from build123d import *

# Parameters (mm, degrees)
SKETCH1_W           = 110
SKETCH1_H           = 48
SKETCH1_R           = 2.1
BOSS_EXTRUDE1_DEPTH = 1.5
FILLET1_R           = 1.5


with BuildPart() as part:
    # Sketch1 → Boss-Extrude1 (new body, symmetric)
    with BuildSketch(Plane.XY):
        Rectangle(SKETCH1_W, SKETCH1_H)
        with Locations((50, 9)):
            Circle(SKETCH1_R, mode=Mode.SUBTRACT)
        with Locations((26, 9)):
            Circle(SKETCH1_R, mode=Mode.SUBTRACT)
        with Locations((50, -9)):
            Circle(SKETCH1_R, mode=Mode.SUBTRACT)
        with Locations((26, -9)):
            Circle(SKETCH1_R, mode=Mode.SUBTRACT)
        with Locations((-50, 9)):
            Circle(SKETCH1_R, mode=Mode.SUBTRACT)
        with Locations((-26, 9)):
            Circle(SKETCH1_R, mode=Mode.SUBTRACT)
        with Locations((-50, -9)):
            Circle(SKETCH1_R, mode=Mode.SUBTRACT)
        with Locations((-26, -9)):
            Circle(SKETCH1_R, mode=Mode.SUBTRACT)
        with Locations((-38, 19.5)):
            Circle(SKETCH1_R, mode=Mode.SUBTRACT)
        with Locations((-38, -19.5)):
            Circle(SKETCH1_R, mode=Mode.SUBTRACT)
        with Locations((38, 19.5)):
            Circle(SKETCH1_R, mode=Mode.SUBTRACT)
        with Locations((38, -19.5)):
            Circle(SKETCH1_R, mode=Mode.SUBTRACT)
        with Locations((12.5, -9)):
            Circle(SKETCH1_R, mode=Mode.SUBTRACT)
        with Locations((-12.5, -9)):
            Circle(SKETCH1_R, mode=Mode.SUBTRACT)
        with Locations((-12.5, 7)):
            Circle(SKETCH1_R, mode=Mode.SUBTRACT)
        with Locations((12.5, 7)):
            Circle(SKETCH1_R, mode=Mode.SUBTRACT)
    extrude(amount=BOSS_EXTRUDE1_DEPTH, both=True)

    # Fillet1
    fillet1_edges = [part.edges().sort_by_distance(p)[0] for p in [
        (-55, 24, 0),
        (55, 24, 0),
        (55, -24, 0),
        (-55, -24, 0),
    ]]
    fillet(fillet1_edges, radius=FILLET1_R)


solid = part.part
The listing builds one solid part. Answer for the finished solid, in the listing's coordinates (mm). Coordinates: 2 decimals unless noted, no trailing zeros. Loops run counter-clockwise (first coordinate to the right, second up) from the corner with the lowest first, then second, coordinate; pieces in that order, holes last. Notation, with made-up numbers: (81.5, 26) -> (106.5, 26) arc R22 ccw to (106.5, 55) -> close; hole circle Ø4 at (19, 32.25). An arc over 180 degrees is marked (long way). Answer in a Markdown table with one row per item. Add a question column.
1. The part is cut by section D-D, the plane z = 0. Count the separate pieces of the cut face and the enclosed holes in it, then the cut area to 3 significant figures.
2. A flat-ended cylindrical pin translates along its axis: P1, Ø3.5, axis at x = 12.5, y = -9, coming from the +Z side. Find the tip coordinate at first contact, or state that the pin passes through.
3. Consider line 1 (Y direction, x = 26, z = 0.85); line 2 (Y direction, x = -12.5, z = 0.7); line 3 (X direction, y = -21, z = -1.2). Determine where each line is inside the solid, lowest interval first. Write a range as [from, to].
4. The part is cut by section C-C, the plane y = -19.5. Write down the section's boundary in (x, z).
5. Determine the mould class of faces 1 (the cylindrical face through (12.227, -6.918, -0.021)), 2 (the flat face through (55, 0, 0)), 3 (the flat face through (-1, 24, 0)), 4 (the cylindrical face through (36.452, -18.081, -0.021)) for opening direction X: +X half, -X half, draft (parallel to the pull), parting line (faces both ways), or undercut.
6. The part is cut by section A-A, the plane y = -9. Write down the section's boundary in (x, z).
7. The part is cut by section B-B, the plane x = -50. Write down the section's boundary in (y, z), then the cut area to 3 significant figures.
Answer below:
| question | item | result |
|---|---|---|
| 1 | separate pieces | 1 |
| 1 | enclosed holes | 16 |
| 1 | area | 5,060 mm2 |
| 2 | P1 | through |
| 3 | line 1 | [-24, -11.1], [-6.9, 6.9], [11.1, 24] |
| 3 | line 2 | [-24, -11.1], [-6.9, 4.9], [9.1, 24] |
| 3 | line 3 | [-55, -39.47], [-36.53, 36.53], [39.47, 55] |
| 4 | outline | (-55, -1.5) -> (-40.1, -1.5) -> (-40.1, 1.5) -> (-55, 1.5) -> close; (-35.9, -1.5) -> (35.9, -1.5) -> (35.9, 1.5) -> (-35.9, 1.5) -> close; (40.1, -1.5) -> (55, -1.5) -> (55, 1.5) -> (40.1, 1.5) -> close |
| 5 | face 1 | undercut |
| 5 | face 2 | +X half |
| 5 | face 3 | draft |
| 5 | face 4 | undercut |
| 6 | outline | (-55, -1.5) -> (-52.1, -1.5) -> (-52.1, 1.5) -> (-55, 1.5) -> close; (-47.9, -1.5) -> (-28.1, -1.5) -> (-28.1, 1.5) -> (-47.9, 1.5) -> close; (-23.9, -1.5) -> (-14.6, -1.5) -> (-14.6, 1.5) -> (-23.9, 1.5) -> close; (-10.4, -1.5) -> (10.4, -1.5) -> (10.4, 1.5) -> (-10.4, 1.5) -> close; (14.6, -1.5) -> (23.9, -1.5) -> (23.9, 1.5) -> (14.6, 1.5) -> close; (28.1, -1.5) -> (47.9, -1.5) -> (47.9, 1.5) -> (28.1, 1.5) -> close; (52.1, -1.5) -> (55, -1.5) -> (55, 1.5) -> (52.1, 1.5) -> close |
| 7 | outline | (-24, -1.5) -> (-11.1, -1.5) -> (-11.1, 1.5) -> (-24, 1.5) -> close; (-6.9, -1.5) -> (6.9, -1.5) -> (6.9, 1.5) -> (-6.9, 1.5) -> close; (11.1, -1.5) -> (24, -1.5) -> (24, 1.5) -> (11.1, 1.5) -> close |
| 7 | area | 119 mm2 |
